```python
from build123d import *

# Parameters (mm, degrees)
SKETCH1_R           = 8.025
BOSS_EXTRUDE1_DEPTH = 16
CUT_EXTRUDE1_START  = -8.55
SKETCH2_R           = 8.025
CUT_EXTRUDE1_DEPTH  = 7.35
SKETCH3_R           = 4
CUT_EXTRUDE2_DEPTH  = 20.616351598
CIRPATTERN1_COUNT   = 2
CIRPATTERN1_ANGLE   = 90


# Read off the part's stored shape, not the designer's step: M3x0.5 Tapped Hole1
with BuildPart() as part:
    # Sketch1 → Boss-Extrude1 (new body)
    with BuildSketch(Plane(origin=(0, 0, 0), x_dir=(1, 0, 0), z_dir=(0, 1, 0))):
        with Locations(Location((0, 0, 0), (0, 0, 270))):
            Circle(SKETCH1_R)
    extrude(amount=BOSS_EXTRUDE1_DEPTH)

    # Sketch2 → Cut-Extrude1 (cut)
    with BuildSketch(Plane(origin=(0, 16, 0), x_dir=(1, 0, 0), z_dir=(0, 1, 0)).offset(CUT_EXTRUDE1_START)):
        with Locations(Location((0, 0, 0), (0, 0, 270))):
            Circle(SKETCH2_R)
        with BuildLine():
            Line((0.223750509, 5.986515514), (0.617084741, 5.197309317))
            ThreePointArc((0.617084741, 5.197309317), (0.801726633, 5.061902746), (1.01917444, 5.133624565))
            Line((1.01917444, 5.133624565), (1.637135651, 5.762657299))
            ThreePointArc((1.637135651, 5.762657299), (1.756034951, 5.830288043), (1.892729091, 5.825221162))
            ThreePointArc((1.892729091, 5.825221162), (2.00629521, 5.748973556), (2.06273441, 5.62437188))
            Line((2.06273441, 5.62437188), (2.192939368, 4.752245221))
            ThreePointArc((2.192939368, 4.752245221), (2.326701311, 4.566408436), (2.555669726, 4.567424872))
            Line((2.555669726, 4.567424872), (3.337767568, 4.974710037))
            ThreePointArc((3.337767568, 4.974710037), (3.471746571, 5.002288793), (3.60018467, 4.955229091))
            ThreePointArc((3.60018467, 4.955229091), (3.684630662, 4.847619447), (3.699803496, 4.711675538))
            Line((3.699803496, 4.711675538), (3.55413381, 3.841998252))
            ThreePointArc((3.55413381, 3.841998252), (3.623922254, 3.623922254), (3.841998252, 3.55413381))
            Line((3.841998252, 3.55413381), (4.711675538, 3.699803496))
            ThreePointArc((4.711675538, 3.699803496), (4.847619447, 3.684630662), (4.955229091, 3.60018467))
            ThreePointArc((4.955229091, 3.60018467), (5.002288793, 3.471746571), (4.974710037, 3.337767568))
            Line((4.974710037, 3.337767568), (4.567424872, 2.555669726))
            ThreePointArc((4.567424872, 2.555669726), (4.566408436, 2.326701311), (4.752245221, 2.192939368))
            Line((4.752245221, 2.192939368), (5.62437188, 2.06273441))
            ThreePointArc((5.62437188, 2.06273441), (5.748973556, 2.00629521), (5.825221162, 1.892729091))
            ThreePointArc((5.825221162, 1.892729091), (5.830288043, 1.756034951), (5.762657299, 1.637135651))
            Line((5.762657299, 1.637135651), (5.133624565, 1.01917444))
            ThreePointArc((5.133624565, 1.01917444), (5.061902746, 0.801726633), (5.197309317, 0.617084741))
            Line((5.197309317, 0.617084741), (5.986515514, 0.223750509))
            ThreePointArc((5.986515514, 0.223750509), (6.087578078, 0.131569604), (6.125, 0))
            ThreePointArc((6.125, 0), (6.087578078, -0.131569604), (5.986515514, -0.223750509))
            Line((5.986515514, -0.223750509), (5.197309317, -0.617084741))
            ThreePointArc((5.197309317, -0.617084741), (5.061902746, -0.801726633), (5.133624565, -1.01917444))
            Line((5.133624565, -1.01917444), (5.762657299, -1.637135651))
            ThreePointArc((5.762657299, -1.637135651), (5.830288043, -1.756034951), (5.825221162, -1.892729091))
            ThreePointArc((5.825221162, -1.892729091), (5.748973556, -2.00629521), (5.62437188, -2.06273441))
            Line((5.62437188, -2.06273441), (4.752245221, -2.192939368))
            ThreePointArc((4.752245221, -2.192939368), (4.566408436, -2.326701311), (4.567424872, -2.555669726))
            Line((4.567424872, -2.555669726), (4.974710037, -3.337767568))
            ThreePointArc((4.974710037, -3.337767568), (5.002288793, -3.471746571), (4.955229091, -3.60018467))
            ThreePointArc((4.955229091, -3.60018467), (4.847619447, -3.684630662), (4.711675538, -3.699803496))
            Line((4.711675538, -3.699803496), (3.841998252, -3.55413381))
            ThreePointArc((3.841998252, -3.55413381), (3.623922254, -3.623922254), (3.55413381, -3.841998252))
            Line((3.55413381, -3.841998252), (3.699803496, -4.711675538))
            ThreePointArc((3.699803496, -4.711675538), (3.684630662, -4.847619447), (3.60018467, -4.955229091))
            ThreePointArc((3.60018467, -4.955229091), (3.471746571, -5.002288793), (3.337767568, -4.974710037))
            Line((3.337767568, -4.974710037), (2.555669726, -4.567424872))
            ThreePointArc((2.555669726, -4.567424872), (2.326701311, -4.566408436), (2.192939368, -4.752245221))
            Line((2.192939368, -4.752245221), (2.06273441, -5.62437188))
            ThreePointArc((2.06273441, -5.62437188), (2.00629521, -5.748973556), (1.892729091, -5.825221162))
            ThreePointArc((1.892729091, -5.825221162), (1.756034951, -5.830288043), (1.637135651, -5.762657299))
            Line((1.637135651, -5.762657299), (1.01917444, -5.133624565))
            ThreePointArc((1.01917444, -5.133624565), (0.801726633, -5.061902746), (0.617084741, -5.197309317))
            Line((0.617084741, -5.197309317), (0.223750509, -5.986515514))
            ThreePointArc((0.223750509, -5.986515514), (0.131569604, -6.087578078), (0, -6.125))
            ThreePointArc((0, -6.125), (-0.131569604, -6.087578078), (-0.223750509, -5.986515514))
            Line((-0.223750509, -5.986515514), (-0.617084741, -5.197309317))
            ThreePointArc((-0.617084741, -5.197309317), (-0.801726633, -5.061902746), (-1.01917444, -5.133624565))
            Line((-1.01917444, -5.133624565), (-1.637135651, -5.762657299))
            ThreePointArc((-1.637135651, -5.762657299), (-1.756034951, -5.830288043), (-1.892729091, -5.825221162))
            ThreePointArc((-1.892729091, -5.825221162), (-2.00629521, -5.748973556), (-2.06273441, -5.62437188))
            Line((-2.06273441, -5.62437188), (-2.192939368, -4.752245221))
            ThreePointArc((-2.192939368, -4.752245221), (-2.326701311, -4.566408436), (-2.555669726, -4.567424872))
            Line((-2.555669726, -4.567424872), (-3.337767568, -4.974710037))
            ThreePointArc((-3.337767568, -4.974710037), (-3.471746571, -5.002288793), (-3.60018467, -4.955229091))
            ThreePointArc((-3.60018467, -4.955229091), (-3.684630662, -4.847619447), (-3.699803496, -4.711675538))
            Line((-3.699803496, -4.711675538), (-3.55413381, -3.841998252))
            ThreePointArc((-3.55413381, -3.841998252), (-3.623922254, -3.623922254), (-3.841998252, -3.55413381))
            Line((-3.841998252, -3.55413381), (-4.711675538, -3.699803496))
            ThreePointArc((-4.711675538, -3.699803496), (-4.847619447, -3.684630662), (-4.955229091, -3.60018467))
            ThreePointArc((-4.955229091, -3.60018467), (-5.002288793, -3.471746571), (-4.974710037, -3.337767568))
            Line((-4.974710037, -3.337767568), (-4.567424872, -2.555669726))
            ThreePointArc((-4.567424872, -2.555669726), (-4.566408436, -2.326701311), (-4.752245221, -2.192939368))
            Line((-4.752245221, -2.192939368), (-5.62437188, -2.06273441))
            ThreePointArc((-5.62437188, -2.06273441), (-5.748973556, -2.00629521), (-5.825221162, -1.892729091))
            ThreePointArc((-5.825221162, -1.892729091), (-5.830288043, -1.756034951), (-5.762657299, -1.637135651))
            Line((-5.762657299, -1.637135651), (-5.133624565, -1.01917444))
            ThreePointArc((-5.133624565, -1.01917444), (-5.061902746, -0.801726633), (-5.197309317, -0.617084741))
            Line((-5.197309317, -0.617084741), (-5.986515514, -0.223750509))
            ThreePointArc((-5.986515514, -0.223750509), (-6.087578078, -0.131569604), (-6.125, 0))
            ThreePointArc((-6.125, 0), (-6.087578078, 0.131569604), (-5.986515514, 0.223750509))
            Line((-5.986515514, 0.223750509), (-5.197309317, 0.617084741))
            ThreePointArc((-5.197309317, 0.617084741), (-5.061902746, 0.801726633), (-5.133624565, 1.01917444))
            Line((-5.133624565, 1.01917444), (-5.762657299, 1.637135651))
            ThreePointArc((-5.762657299, 1.637135651), (-5.830288043, 1.756034951), (-5.825221162, 1.892729091))
            ThreePointArc((-5.825221162, 1.892729091), (-5.748973556, 2.00629521), (-5.62437188, 2.06273441))
            Line((-5.62437188, 2.06273441), (-4.752245221, 2.192939368))
            ThreePointArc((-4.752245221, 2.192939368), (-4.566408436, 2.326701311), (-4.567424872, 2.555669726))
            Line((-4.567424872, 2.555669726), (-4.974710037, 3.337767568))
            ThreePointArc((-4.974710037, 3.337767568), (-5.002288793, 3.471746571), (-4.955229091, 3.60018467))
            ThreePointArc((-4.955229091, 3.60018467), (-4.847619447, 3.684630662), (-4.711675538, 3.699803496))
            Line((-4.711675538, 3.699803496), (-3.841998252, 3.55413381))
            ThreePointArc((-3.841998252, 3.55413381), (-3.623922254, 3.623922254), (-3.55413381, 3.841998252))
            Line((-3.55413381, 3.841998252), (-3.699803496, 4.711675538))
            ThreePointArc((-3.699803496, 4.711675538), (-3.684630662, 4.847619447), (-3.60018467, 4.955229091))
            ThreePointArc((-3.60018467, 4.955229091), (-3.471746571, 5.002288793), (-3.337767568, 4.974710037))
            Line((-3.337767568, 4.974710037), (-2.555669726, 4.567424872))
            ThreePointArc((-2.555669726, 4.567424872), (-2.326701311, 4.566408436), (-2.192939368, 4.752245221))
            Line((-2.192939368, 4.752245221), (-2.06273441, 5.62437188))
            ThreePointArc((-2.06273441, 5.62437188), (-2.00629521, 5.748973556), (-1.892729091, 5.825221162))
            ThreePointArc((-1.892729091, 5.825221162), (-1.756034951, 5.830288043), (-1.637135651, 5.762657299))
            Line((-1.637135651, 5.762657299), (-1.01917444, 5.133624565))
            ThreePointArc((-1.01917444, 5.133624565), (-0.801726633, 5.061902746), (-0.617084741, 5.197309317))
            Line((-0.617084741, 5.197309317), (-0.223750509, 5.986515514))
            ThreePointArc((-0.223750509, 5.986515514), (-0.131569604, 6.087578078), (0, 6.125))
            ThreePointArc((0, 6.125), (0.131569604, 6.087578078), (0.223750509, 5.986515514))
        make_face(mode=Mode.SUBTRACT)
    extrude(amount=CUT_EXTRUDE1_DEPTH, mode=Mode.SUBTRACT)

    # Sketch3 → Cut-Extrude2 (cut, through all)
    with BuildSketch(Plane(origin=(0, 16, 0), x_dir=(1, 0, 0), z_dir=(0, 1, 0))):
        with Locations(Location((0, 0, 0), (0, 0, 270))):
            Circle(SKETCH3_R)
    extrude(amount=-CUT_EXTRUDE2_DEPTH, mode=Mode.SUBTRACT)

    # M3x0.5 Tapped Hole1 outline → M3x0.5 Tapped Hole1 (revolve, cut)
    with BuildSketch(Plane.XZ.offset(-3.725)):
        Polygon((2.000000319, 8.025000319), (0, 8.025000319), (0, 3.799586083), (1.25, 3.799586083), (1.25, 7.275), align=None)
    m3x0_5_tapped_hole1 = revolve(axis=Axis((0, 3.725, 0), (0, 0, 1)), mode=Mode.SUBTRACT)

    # CirPattern1: M3x0.5 Tapped Hole1 ×2 about axis
    cirpattern1_axis = Axis((0, 16, 0), (0, 1, 0))
    for i in range(1, CIRPATTERN1_COUNT):
        add(m3x0_5_tapped_hole1.rotate(cirpattern1_axis, i * CIRPATTERN1_ANGLE / (CIRPATTERN1_COUNT - 1)), mode=Mode.SUBTRACT)


solid = part.part
```
Check sheet for the modelled part. Datum: model origin and axes. Units: mm. A direction names the side the tool comes from. Give positions to 0.01 mm unless a question says otherwise; leave off trailing zeros. Loops run counter-clockwise (first coordinate to the right, second up) from the corner with the lowest first, then second, coordinate; pieces in that order, holes last. Notation, with made-up numbers: M -37.75,-11 L 8.25,-11 A18 ccw 8.25,9 Z; hole C 4.25,58 d1. An arc over 180 degrees is marked long. Answer in a Markdown table with one row per item.
1) Cross-section at A-A (x = -6.5). Enter the section's corners in (y, z).
Solutions:
| item | result |
|---|---|
| outline | M 0,-4.71 L 7.45,-4.71 L 7.45,4.71 L 0,4.71 Z; M 14.8,-4.71 L 16,-4.71 L 16,4.71 L 14.8,4.71 Z |
2) Mould release check, pull along X, two halves, no side actions. Record for faces 1 (the face through (-5.18, 11.07, 2.13)), 2 (the face through (-0.271, 2.505, 5.562)), 3 (the face through (-3.905, 8.112, -0.867)), 4 (the face through (5.559, 2.505, 0.271)): released by +X, released by -X, zero draft, split by the parting line, or undercut.
Solutions:
| item | result |
|---|---|
| face 1 | released by -X |
| face 2 | undercut |
| face 3 | undercut |
| face 4 | zero draft |
3) Tool access check on faces 5 (the face through (5, 14.8, 3)), 6 (the face through (2.127, 11.074, -5.194)), 7 (the face through (-4.271, 11.074, 3.626)), 8 (the face through (-3.626, 11.074, -4.271)), 9 (the face through (3.628, 11.074, -4.283)). Record the directions out of +Z, -Z, +X, -X, +Y, -Y that give a thin tool (end or side, any length) a straight path to the whole face; none if there is none.
Solutions:
| item | result |
|---|---|
| face 5 | none |
| face 6 | -Z |
| face 7 | +Z |
| face 8 | -X |
| face 9 | +X |
4) Thickness scan on line 1 (Y direction, x = 0, z = 6.4) (3 decimals); line 2 (Z direction, x = -1.5, y = 9.5); line 3 (Y direction, x = 5.4, z = 0) (3 decimals). Record the ranges inside material, lowest first.
Solutions:
| item | result |
|---|---|
| line 1 | y = 0 to 2.475, 4.975 to 7.45, 14.8 to 16 |
| line 2 | z = -5.62 to -3.71, 3.71 to 5.62 |
| line 3 | y = 0 to 2.475, 4.975 to 16 |
5) Depth check by flat-ended pin: pin 1 (5 mm diameter, centred on x = 0, z = 0, fed in from -Y); pin 2 (3 mm diameter, centred on x = 4.5, y = 7.5, fed in from -Z); pin 3 (3 mm diameter, centred on y = 12, z = 2.5, fed in from +X). Enter the tip coordinate at first touch or a pass-through.
Solutions:
| item | result |
|---|---|
| pin 1 | passes through |
| pin 2 | stops at z = -7.44 |
| pin 3 | stops at x = 5.84 |
